The model under review builds one solid part; all positions refer to its coordinate system, in mm. A direction names the side the tool comes from. Coordinates: 2 decimals unless noted, no trailing zeros. Loops run counter-clockwise (first coordinate to the right, second up) from the corner with the lowest first, then second, coordinate; pieces in that order, holes last. Notation, with made-up numbers: (4.25, 69) - (36.25, 69) arc R15 ccw to (36.25, 97) - close; hole circle Ø11 at (33.25, -35). An arc over 180 degrees is marked (long way). One line per item, written item: value. Start each with the question number.
1. We need section A-A, the plane x = 0. Give the boundary of the cut face in (y, z), then the cut area to 3 significant figures.
2. We need section C-C, the plane y = -0.8. Give the boundary of the cut face in (x, z).
3. Insertion check: P1, Ø1, axis at x = 0, z = 15.5, coming from the -Y side; P2, Ø0.6, axis at x = 0, z = 16.5, coming from the +Y side; P3, Ø2, axis at x = 2, z = 54, coming from the +Y side. Each pin has a flat end and moves straight along its axis. Give the tip position at first contact, or say it passes through.
4. For faces 1 (the face through (1.49, -0.88, 15.97)), 2 (the face through (-1.51, -0.85, 5.97)), 3 (the face through (1.51, 0.85, 15.97)), list the 3-axis set-ups (+Z, -Z, +X, -X, +Y, -Y) from which the entire face can be reached by the end or side of a thin tool; tool diameter is ignored.
5. We need section B-B, the plane z = 47.5. Give the boundary of the cut face in (x, y), then the cut area to 3 significant figures.
6. To check wall thickness, follow line 1 (Z direction, x = 2.45, y = 0.3); line 2 (Y direction, x = -0.3, z = 15.5); line 3 (Y direction, x = -1.55, z = 36.5). State the ranges of each line that lie inside material, in increasing order.
7. Mouldability with a two-part tool opening along Z and no side actions: class faces 4 (the face through (-1.49, 0.88, 15.97)), 5 (the face through (-2.262, -1.734, 46.298)), 6 (the face through (0, 0, 0)) as +Z half, -Z half, draft (parallel to the pull), parting line (faces both ways), or undercut.
from build123d import *

# Parameters (mm, degrees)
SKETCH_1_R      = 2.85
EXTRUDE_1_DEPTH = 4
EXTRUDE_2_DEPTH = 4
SKETCH_3_R      = 2.85
EXTRUDE_3_DEPTH = 6
EXTRUDE_4_DEPTH = 4
SKETCH_6_R      = 2.85
EXTRUDE_5_DEPTH = 57.4


with BuildPart() as part:
    # 草图1 → 凸台-拉伸1 (new body)
    with BuildSketch(Plane.XY):
        Circle(SKETCH_1_R)
    extrude(amount=EXTRUDE_1_DEPTH)

    # 草图2 → 凸台-拉伸2 (add)
    with BuildSketch(Plane.XY.offset(4)):
        Polygon((2, 0), (1, 1.732050808), (-1, 1.732050808), (-2, 0), (-1, -1.732050808), (1, -1.732050808), align=None)
    extrude(amount=EXTRUDE_2_DEPTH)

    # 草图3 → 凸台-拉伸3 (add)
    with BuildSketch(Plane.XY.offset(8)):
        Circle(SKETCH_3_R)
    extrude(amount=EXTRUDE_3_DEPTH)

    # 草图4 → 凸台-拉伸4 (add)
    with BuildSketch(Plane.XY.offset(14)):
        Polygon((2, 0), (1, 1.732050808), (-1, 1.732050808), (-2, 0), (-1, -1.732050808), (1, -1.732050808), align=None)
    extrude(amount=EXTRUDE_4_DEPTH)

    # 草图6 → 凸台-拉伸5 (add)
    with BuildSketch(Plane.XY.offset(18)):
        Circle(SKETCH_6_R)
    extrude(amount=EXTRUDE_5_DEPTH)


solid = part.part
Findings below:
1. outline: (-2.85, 0) - (2.85, 0) - (2.85, 4) - (1.73, 4) - (1.73, 8) - (2.85, 8) - (2.85, 14) - (1.73, 14) - (1.73, 18) - (2.85, 18) - (2.85, 75.4) - (-2.85, 75.4) - (-2.85, 18) - (-1.73, 18) - (-1.73, 14) - (-2.85, 14) - (-2.85, 8) - (-1.73, 8) - (-1.73, 4) - (-2.85, 4) - close
1. area: 412 mm2
2. outline: (-2.74, 0) - (2.74, 0) - (2.74, 4) - (1.54, 4) - (1.54, 8) - (2.74, 8) - (2.74, 14) - (1.54, 14) - (1.54, 18) - (2.74, 18) - (2.74, 75.4) - (-2.74, 75.4) - (-2.74, 18) - (-1.54, 18) - (-1.54, 14) - (-2.74, 14) - (-2.74, 8) - (-1.54, 8) - (-1.54, 4) - (-2.74, 4) - close
3. P1: y = -1.73
3. P2: y = 1.73
3. P3: y = 2.67
4. face 1: +X, -Y
4. face 2: -X, -Y
4. face 3: +X, +Y
5. outline: circle Ø5.7 at (0, 0)
5. area: 25.5 mm2
6. line 1: 0 to 4, 8 to 14, 18 to 75.4
6. line 2: -1.73 to 1.73
6. line 3: -2.39 to 2.39
7. face 4: undercut
7. face 5: draft
7. face 6: -Z half
